Geometry: see drawing. Coordinates: mm, zero at the bounding-box minimum. Give positions to 0.01 mm unless a question says otherwise; leave off trailing zeros. Write each loop counter-clockwise with the first axis right and the second up, starting at its lowest first coordinate (ties: lowest second). Pieces come first, ordered by that corner, then holes. Notation, with made-up numbers: (32, -16.5) -> (79, -16.5) arc R23 ccw to (79, 1.5) -> close; hole circle Ø1 at (66, 25.5). An arc over 180 degrees is marked (long way). Answer as a JSON object with one key per item and string values. Group by question number.
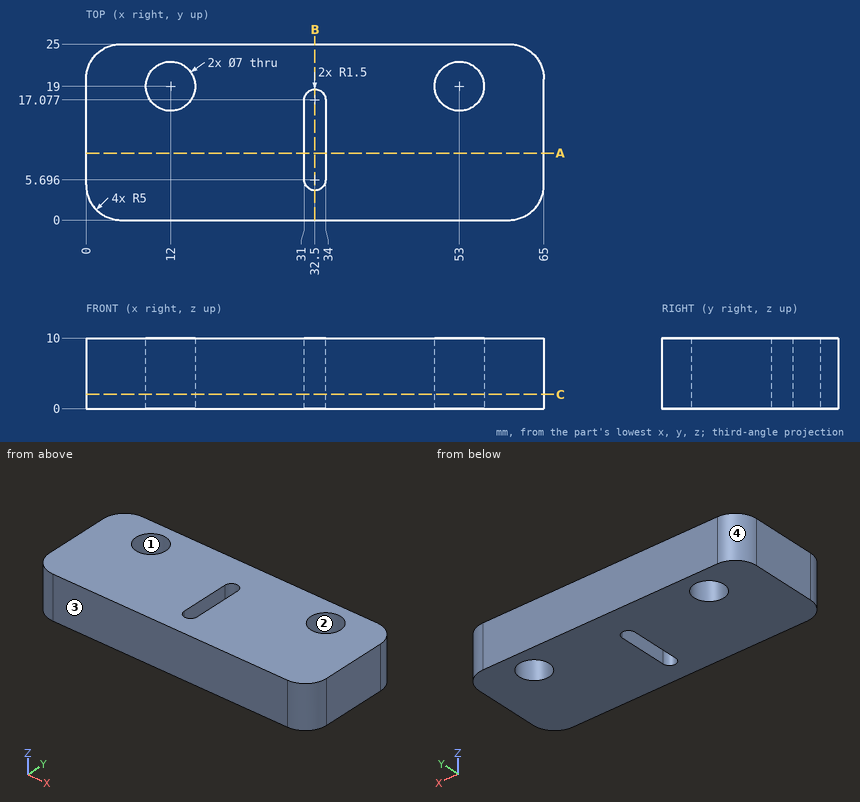
1. Section A-A (y = 9.5). Return the cut outline in (x, z), plus the area to 3 significant figures.
2. Section C-C (z = 2). Return the cut outline in (x, y), plus the area to 3 significant figures.
3. Mould query, pull axis Y, two halves, no side actions, for the marked faces 1, 2, 3 and 4. Classes: pulls with the +Y half, pulls with the -Y half, needs draft (parallel to the pull), parting line crosses it, or undercut.
4. Line query: line 1 (X direction, y = 12.25, z = 8.25); line 2 (Y direction, x = 53, z = 2); line 3 (X direction, y = 20.25, z = 9). Output: solid intervals per line, ascending.
5. Section B-B (x = 32.5). Return the cut outline in (y, z), plus the area to 3 significant figures.
Working result:
{
 "1": {"outline": "(0, 0) -> (31, 0) -> (31, 10) -> (0, 10) -> close; (34, 0) -> (65, 0) -> (65, 10) -> (34, 10) -> close", "area": "620 mm^2"},
 "2": {"outline": "(0, 5) arc R5 ccw to (5, 0) -> (60, 0) arc R5 ccw to (65, 5) -> (65, 20) arc R5 ccw to (60, 25) -> (5, 25) arc R5 ccw to (0, 20) -> close; hole circle Ø7 at (12, 19); hole (31, 5.7) arc R1.5 ccw to (34, 5.7) -> (34, 17.08) arc R1.5 ccw to (31, 17.08) -> close; hole circle Ø7 at (53, 19)", "area": "1,490 mm^2"},
 "3": {"face 1": "undercut", "face 2": "undercut", "face 3": "pulls with the -Y half", "face 4": "pulls with the +Y half"},
 "4": {"line 1": "x = 0 to 31, 34 to 65", "line 2": "y = 0 to 15.5, 22.5 to 25", "line 3": "x = 0.01 to 8.73, 15.27 to 49.73, 56.27 to 64.99"},
 "5": {"outline": "(0, 0) -> (4.2, 0) -> (4.2, 10) -> (0, 10) -> close; (18.58, 0) -> (25, 0) -> (25, 10) -> (18.58, 10) -> close", "area": "106 mm^2"}
}
